Could you check a few things on this drawing? It's one solid part, dimensions in mm from its lowest x, y, z. A direction names the side the tool comes from. Round coordinates to 2 decimals unless told otherwise and drop trailing zeros. Loops run counter-clockwise (first coordinate to the right, second up) from the corner with the lowest first, then second, coordinate; pieces in that order, holes last. Notation, with made-up numbers: M 3.5,31.25 L 47.5,31.25 A18 ccw 47.5,59.25 Z; hole C 73,33.25 d1. An arc over 180 degrees is marked long. Return JSON: item names as keys, results as strings.
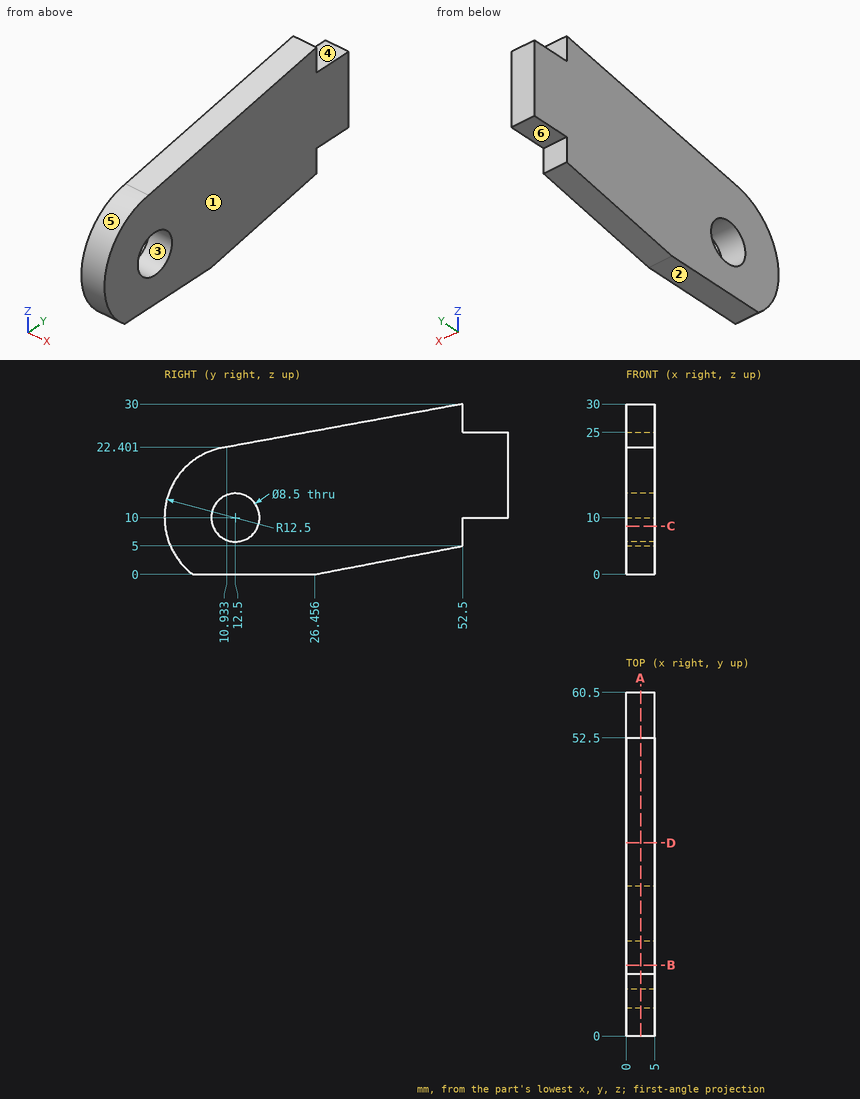
Q1. On a 3-axis mill with a long thin cutter (end or side, diameter ignored), from which of +Z, -Z, +X, -X, +Y, -Y can I reach the whole of each face in a straight line? I mean the marked faces 4, 5 and 6. Say none if no direction works.
Results:
{"face 4": "+Z, +X, -X, +Y", "face 5": "+X, -X, -Y", "face 6": "-Z, +X, -X, +Y"}
Q2. Suppose I cut it at D-D, the plane y = 34. Please give me the cut outline in (x, z).
Results:
{"outline": "M 0,1.45 L 5,1.45 L 5,26.62 L 0,26.62 Z"}
Q3. Suppose I cut it at B-B, the plane y = 12.5. Please give me the cut outline in (x, z).
Results:
{"outline": "M 0,0 L 5,0 L 5,5.75 L 0,5.75 Z; M 0,14.25 L 5,14.25 L 5,22.69 L 0,22.69 Z"}
Q4. Thinking about a two-plate mould opening in Z: for the marked faces 1, 2 and 3, which applies, pulls with the +Z half, pulls with the -Z half, needs draft (parallel to the pull), parting line crosses it, or undercut?
Results:
{"face 1": "needs draft", "face 2": "pulls with the -Z half", "face 3": "undercut"}
Q5. I'm going to push flat-ended pins straight in: pin 1 Ø2.5 at (x, z) = (2, 27.5) entering from +Y; pin 2 Ø2.5 at (x, y) = (3.5, 57) entering from +Z; pin 3 Ø1.5 at (x, y) = (2.5, 42) entering from -Z. Where does each tip first touch, or does it pass through?
Results:
{"pin 1": "stops at y = 52.5", "pin 2": "stops at z = 25", "pin 3": "stops at z = 2.84"}
Q6. Suppose I cut it at C-C, the plane z = 8.5. Please give me the cut outline in (x, y).
Results:
{"outline": "M 0,0.09 L 5,0.09 L 5,8.52 L 0,8.52 Z; M 0,16.48 L 5,16.48 L 5,52.5 L 0,52.5 Z"}
Q7. Suppose I cut it at A-A, the plane x = 2.55. Please give me the cut outline in (y, z).
Results:
{"outline": "M 5,0 L 26.46,0 L 52.5,5 L 52.5,10 L 60.5,10 L 60.5,25 L 52.5,25 L 52.5,30 L 10.93,22.4 A12.5 ccw Z; hole C 12.5,10 d8.5"}
Q8. If I drill on line 1 along Z through (x, y) = (4.05, 12.5); line 2 along Y through (x, z) = (3.6, 19) (1 decimal); line 3 along Y through (x, z) = (0.5, 21.5) (1 decimal), over which ranges is the centre line in solid material (lowest first)?
Results:
{"line 1": "z = 0 to 5.75, 14.25 to 22.69", "line 2": "y = 3.8 to 60.5", "line 3": "y = 7.6 to 60.5"}
